```python
from build123d import *

# Parameters (mm, degrees)
F1_DEPTH = 88.9
F3_DEPTH = 76.201


with BuildPart() as f1:
    # F0 (on Front) → F1 (new body)
    with BuildSketch(Plane.XZ):
        Polygon((0, 61.038002), (0, 0), (76.2, 0), (76.2, 50.8), (66.04, 61.038002), align=None)
        Polygon((0, 67.31), (0, 61.038002), (66.04, 61.038002), (50.8, 67.31), align=None)
    extrude(amount=F1_DEPTH)

    # F2 (on face) → F3 (cut, through all)
    with BuildSketch(Plane(origin=(0, 0, 0), x_dir=(0, -1, 0), z_dir=(-1, 0, 0))):
        with BuildLine():
            ThreePointArc((6.35, 15.875), (24.500933, 6.638738), (44.45, 2.54))
            ThreePointArc((44.45, 2.54), (64.399067, 6.638738), (82.55, 15.875))
            Line((82.55, 15.875), (82.55, 33.655))
            Line((82.55, 33.655), (82.55, 46.355))
            ThreePointArc((82.55, 46.355), (65.0875, 58.1025), (44.45, 62.23))
            ThreePointArc((44.45, 62.23), (23.8125, 58.1025), (6.35, 46.355))
            Line((6.35, 46.355), (6.35, 33.655))
            Line((6.35, 33.655), (6.35, 15.875))
        make_face()
    extrude(amount=-F3_DEPTH, mode=Mode.SUBTRACT)


solid = f1.part
```
Source: CAD feature listing. Evaluate the final solid. Frame: model axes, mm. A direction names the side the tool comes from. Round coordinates to 2 decimals unless told otherwise and drop trailing zeros. Write each loop counter-clockwise with the first axis right and the second up, starting at its lowest first coordinate (ties: lowest second). Pieces come first, ordered by that corner, then holes. Notation, with made-up numbers: M 78,68 L 96,68 A21 ccw 96,78 Z; hole C 64.25,42.25 d5. An arc over 180 degrees is marked long. Use CSV: the item, a comma, the result in double quotes. Start each with the question number.
Q1. Cut plane B-B on z = 22. Output: boundary loops of the cut face in (x, y), plus the area to 3 significant figures.
Q2. Cut plane C-C on y = -68. Output: boundary loops of the cut face in (x, z), plus the area to 3 significant figures.
Q3. First-contact query: P1, Ø4, axis at x = 12, z = 18.5, coming from the +Y side; P2, Ø3, axis at x = 56.5, y = -71, coming from the +Z side. Flat tips, straight axial feed; report the tip coordinate or a pass-through.
Q4. Pull-direction query (Y, two-part tool) for faces 3 (the face through (38, 0, 34)), 4 (the face through (58.53, -43.83, 64.13)), 5 (the face through (38, -6.35, 31)); classes: +Y half, -Y half, draft (parallel to the pull), parting line (faces both ways), or undercut.
Q5. Cut plane D-D on z = 9.5. Output: boundary loops of the cut face in (x, y).
Q6. Line query: line 1 (Y direction, x = 60, z = 18); line 2 (Z direction, x = 17, y = -43). Output: solid intervals per line, ascending. Write a range as from..to.
Q7. Access query for faces 1 (the face through (37.567, -45.043, 62.227)), 2 (the face through (38, -44, 0)). Directions: +Z, -Z, +X, -X, +Y, -Y. A direction counts if a zero-diameter tool reaches every point of the face in a straight line with its end or side. Return the directions, or none.
Results found:
1,outline,"M 0,-88.9 L 76.2,-88.9 L 76.2,-82.55 L 0,-82.55 Z; M 0,-6.35 L 76.2,-6.35 L 76.2,0 L 0,0 Z"
1,area,"968 mm^2"
2,outline,"M 0,0 L 76.2,0 L 76.2,8 L 0,8 Z; M 0,56.79 L 70.26,56.79 L 66.04,61.04 L 50.8,67.31 L 0,67.31 Z"
2,area,"1,270 mm^2"
3,P1,"y = 0"
3,P2,"z = 65.58"
4,face 3,"+Y half"
4,face 4,"draft"
4,face 5,"undercut"
5,outline,"M 0,-88.9 L 76.2,-88.9 L 76.2,-71.43 L 0,-71.43 Z; M 0,-17.47 L 76.2,-17.47 L 76.2,0 L 0,0 Z"
6,line 1,"-88.9..-82.55, -6.35..0"
6,line 2,"0..2.65, 62.21..67.31"
7,face 1,"+X, -X"
7,face 2,"-Z, +X, -X, +Y, -Y"
